from build123d import *

# Parameters (mm, degrees)
BOSS_EXTRUDE1_DEPTH = 205
CUT_EXTRUDE3_DEPTH  = 38.907676661
SKETCH5_W           = 20
SKETCH5_H           = 5
SKETCH5_W_2         = 3
SKETCH5_H_2         = 20
SKETCH5_H_3         = 3
BOSS_EXTRUDE2_DEPTH = 5


with BuildPart() as part:
    # Sketch2 → Boss-Extrude1 (new body)
    with BuildSketch(Plane.XY.offset(14.2)):
        Polygon((-52.961538618, -36.862052104), (-51.252736373, -41.56098761), (-147.541457764, -76.577085001), (-149.250260009, -71.878149495), align=None)
    extrude(amount=BOSS_EXTRUDE1_DEPTH)

    # Sketch4 → Cut-Extrude3 (cut, through all)
    with BuildSketch(Plane(origin=(7.362313595, -20.245196221, 0), x_dir=(-0.939787101, -0.341760449, 0), z_dir=(0.341760449, -0.939787101, 0))):
        Polygon((111.499570088, -14.2), (115.699570088, -14.2), (115.699570088, -18.2), (117.399570088, -18.2), (117.399570088, -21), (115.699570088, -21), (115.699570088, -31), (111.499570088, -31), (111.499570088, -21), (109.799570088, -21), (109.799570088, -18.2), (111.499570088, -18.2), align=None)
        Polygon((62.37056233, -67.55), (62.37056233, -63.35), (66.37056233, -63.35), (66.37056233, -61.65), (69.17056233, -61.65), (69.17056233, -63.35), (79.17056233, -63.35), (79.17056233, -67.55), (69.17056233, -67.55), (69.17056233, -69.25), (66.37056233, -69.25), (66.37056233, -67.55), align=None)
        Polygon((115.699570088, -219.2), (111.499570088, -219.2), (111.499570088, -215.2), (109.799570088, -215.2), (109.799570088, -212.4), (111.499570088, -212.4), (111.499570088, -202.4), (115.699570088, -202.4), (115.699570088, -212.4), (117.399570088, -212.4), (117.399570088, -215.2), (115.699570088, -215.2), align=None)
        Polygon((66.37056233, -170.05), (66.37056233, -171.75), (69.17056233, -171.75), (69.17056233, -170.05), (79.17056233, -170.05), (79.17056233, -165.85), (69.17056233, -165.85), (69.17056233, -164.15), (66.37056233, -164.15), (66.37056233, -165.85), (62.37056233, -165.85), (62.37056233, -170.05), align=None)
        Polygon((164.828577846, -165.85), (164.828577846, -170.05), (160.828577846, -170.05), (160.828577846, -171.75), (158.028577846, -171.75), (158.028577846, -170.05), (148.028577846, -170.05), (148.028577846, -165.85), (158.028577846, -165.85), (158.028577846, -164.15), (160.828577846, -164.15), (160.828577846, -165.85), align=None)
        Polygon((160.828577846, -63.35), (160.828577846, -61.65), (158.028577846, -61.65), (158.028577846, -63.35), (148.028577846, -63.35), (148.028577846, -67.55), (158.028577846, -67.55), (158.028577846, -69.25), (160.828577846, -69.25), (160.828577846, -67.55), (164.828577846, -67.55), (164.828577846, -63.35), align=None)
    extrude(amount=-CUT_EXTRUDE3_DEPTH, mode=Mode.SUBTRACT)

    # Sketch5 → Boss-Extrude2 (add)
    with BuildSketch(Plane(origin=(7.362313595, -20.245196221, 0), x_dir=(0.939787101, 0.341760449, 0), z_dir=(0.341760449, -0.939787101, 0))):
        with Locations((-86.935066209, 11.7)):
            Rectangle(SKETCH5_W, SKETCH5_H)
        with Locations((-140.264073967, 11.7)):
            Rectangle(SKETCH5_W, SKETCH5_H)
        with Locations((-60.87056233, 116.7)):
            Rectangle(SKETCH5_W_2, SKETCH5_H_2)
        with Locations((-60.87056233, 194.625)):
            Rectangle(SKETCH5_W_2, SKETCH5_H_2)
        with Locations((-86.935066209, 220.7)):
            Rectangle(SKETCH5_W, SKETCH5_H_3)
        with Locations((-140.264073967, 220.7)):
            Rectangle(SKETCH5_W, SKETCH5_H_3)
    extrude(amount=-BOSS_EXTRUDE2_DEPTH)


solid = part.part
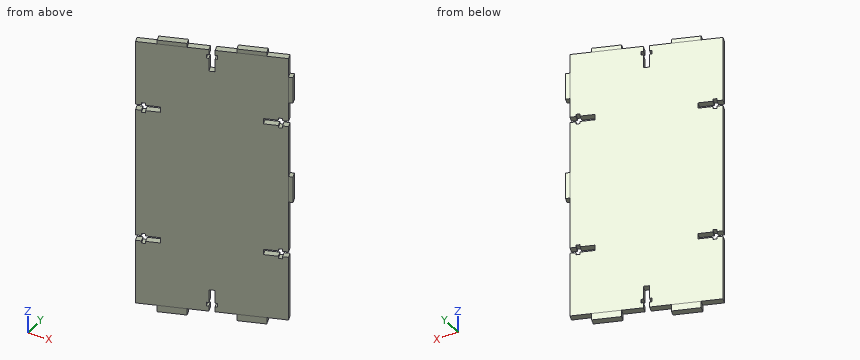
Build history of the part. All positions in model axes, mm. Round coordinates to 2 decimals unless told otherwise and drop trailing zeros. Write each loop counter-clockwise with the first axis right and the second up, starting at its lowest first coordinate (ties: lowest second). Pieces come first, ordered by that corner, then holes. Notation, with made-up numbers: (43.25, 11.5) - (98.25, 11.5) arc R27 cw to (98.25, 37.5) - close; hole circle Ø10 at (57.25, -17.5). An arc over 180 degrees is marked (long way). One line per question, with ' | ' between items.
1. Band-saw the part on B-B, the plane y = -51. Write the cut outline in (x, z).
Results are:
outline: (-91.84, 14.2) - (-84.6, 14.2) - (-84.6, 9.2) - (-77.21, 9.2) - (-77.21, 222.2) - (-84.6, 222.2) - (-84.6, 219.2) - (-91.84, 219.2) - close
2. Band-saw the part on D-D, the plane x = -108. Write the cut outline in (y, z), and give its area (3 significant figures).
Results are:
outline: (-62.2, 14.2) - (-56.88, 14.2) - (-56.88, 219.2) - (-62.2, 219.2) - close | area: 1,090 mm^2
3. Drop flat-ended pins along their axis: pin 1 Ø2 at (x, y) = (-144, -72.5) entering from -Z; pin 2 Ø3 at (x, z) = (-130.5, 170) entering from +Y; pin 3 Ø4 at (x, z) = (-120, 148.5) entering from -Y. Give the stop position or say it passes through.
Results are:
pin 1: z = 14.2 | pin 2: y = -64.51 | pin 3: y = -67.29
4. Band-saw the part on C-C, the plane z = 134. Write the cut outline in (x, y).
Results are:
outline: (-149.25, -71.88) - (-147.54, -76.58) - (-51.25, -41.56) - (-52.96, -36.86) - close
5. Band-saw the part on A-A, the plane x = -120.5. Write the cut outline in (y, z), and give its area (3 significant figures).
Results are:
outline: (-66.74, 9.2) - (-61.42, 9.2) - (-61.42, 222.2) - (-66.74, 222.2) - close | area: 1,130 mm^2
6. Drill centre lines: line 1 along Z through (x, y) = (-136, -69.5); line 2 along Y through (x, z) = (-93.5, 99.5); line 3 along Y through (x, z) = (-126, 179). Where is each one in solid material? Low to high. Write a range as from..to.
Results are:
line 1: 14.2..63.35, 67.55..165.85, 170.05..219.2 | line 2: -56.92..-51.6 | line 3: -68.74..-63.42
